For this review, take the finished solid that the model builds, in its own axes (mm). A direction names the side the tool comes from. Give positions to 0.01 mm unless a question says otherwise; leave off trailing zeros. Order: outer loops, then holes, each group sorted by start corner. A loop starts at its lowest first (then second) coordinate and runs counter-clockwise, first axis right, second up. Notation, with made-up numbers: (32, -16.75) - (51, -16.75) arc R8 cw to (51, -10.75) - close; hole circle Ø3 at (60.25, 38). An arc over 180 degrees is marked (long way). One line per item, written item: value.
```python
from build123d import *

# Parameters (mm, degrees)
F2_R     = 0.5
F3_SIZE  = 0.5
F5_DEPTH = 2.38


# Not quite as in the source:
# - a fillet or chamfer that OpenCascade refuses, or shapes differently, is made with other operations: its cross-section is extruded or revolved along the edge and cut away or added


with BuildPart() as f1:
    # F0 (on Front) → F1 (revolve)
    with BuildSketch(Plane.XZ):
        Polygon((-3, 0), (0, 0), (0, 18), (-1.5, 18.8660254038), (-1.5, 24), (-5, 24), (-5, 20), (-3, 20), (-3, 14.25), (-2.5, 14), (-3, 13.75), align=None)
    revolve(axis=Axis((0, 0, 18.332445994), (0, 0, 1)))

    # F2
    f2_edges = [f1.edges().sort_by_distance(p)[0] for p in [
        (5, 0, 24),
    ]]
    fillet(f2_edges, radius=F2_R)

    # F3
    f3_edges = [f1.edges().sort_by_distance(p)[0] for p in [
        (3, 0, 0),
    ]]
    chamfer(f3_edges, length=F3_SIZE)

    # F4 (on face) → F5 (cut)
    with BuildSketch(Plane.XY.offset(24)):
        Polygon((-1.443375673, -2.5), (1.443375673, -2.5), (2.8867513459, 0), (1.443375673, 2.5), (-1.443375673, 2.5), (-2.8867513459, 0), align=None)
    extrude(amount=-F5_DEPTH, mode=Mode.SUBTRACT)

    # F6: chamfer of 1 x 1.7320508076 on 1 edges, made by hand


with BuildPart() as f6_tool2:
    # F6_s3 → F6_t4 (revolve)
    with BuildSketch(Plane.XZ):
        Polygon((-3.2320508076, 21.62), (-1.5, 20.62), (-1.5, 21.62), align=None)
    revolve(axis=Axis((0, 0, 21.62), (0, 0, 1)))

    split(bisect_by=Plane(origin=(-2.1650635095, 1.25, 0), x_dir=(0, 0, 1), z_dir=(0.8660254038, -0.5, 0)), keep=Keep.TOP)

    split(bisect_by=Plane.XZ.offset(-2.5), keep=Keep.TOP)

    split(bisect_by=Plane(origin=(2.1650635095, 1.25, 0), x_dir=(0, 0, 1), z_dir=(-0.8660254038, -0.5, 0)), keep=Keep.TOP)

    split(bisect_by=Plane(origin=(2.1650635095, -1.25, 0), x_dir=(0, 0, 1), z_dir=(-0.8660254038, 0.5, 0)), keep=Keep.TOP)

    split(bisect_by=Plane.XZ.offset(2.5), keep=Keep.BOTTOM)

    split(bisect_by=Plane(origin=(-2.1650635095, -1.25, 0), x_dir=(0, 0, 1), z_dir=(0.8660254038, 0.5, 0)), keep=Keep.TOP)


with BuildPart() as f1_1:
    add(f1.part)

    # F6_t1: cut F6_tool2
    add(f6_tool2.part, mode=Mode.SUBTRACT)


solid = f1_1.part
```
(1) Draft analysis for pull direction Y (two halves, no side actions). For faces 4 (the face through (3, 0, 17)), 5 (the face through (-3.3, -0.1, 20)), 6 (the face through (1.5, -0.07, 19.76)), state which applies: pulls with the +Y half, pulls with the -Y half, needs draft (parallel to the pull), parting line crosses it, or undercut.
Answers below:
face 4: parting line crosses it
face 5: needs draft
face 6: undercut
(2) Machinability: for faces 1 (the face through (0, 2.5, 23)), 2 (the face through (3, 0, 7)), 3 (the face through (2, 2, 24)), which of the approach directions +Z, -Z, +X, -X, +Y, -Y give a long, thin tool a straight path to every point of the face, cutting with its end or side? Answer none if there is none.
Answers below:
face 1: +Z
face 2: -Z
face 3: +Z, +X, -X, +Y, -Y
(3) Wall thickness on line 1 (X direction, y = 0, z = 19.65); line 2 (Y direction, x = 0, z = 20.25): over which ranges is each line inside the solid? List them lowest first. Write a range as from..to.
Answers below:
line 1: x = -3..-1.5, 1.5..3
line 2: y = -5..-1.5, 1.5..5
(4) Take a section at A-A (z = 11.5). Write out the cut boundary in (x, y), then the cut area to 3 significant figures.
Answers below:
outline: circle Ø6 at (0, 0)
area: 28.3 mm^2
(5) For P1, Ø0.8, axis at x = 0.5, z = 23, coming from the -Y side; P2, Ø3, axis at x = 3.5, z = 15.5, coming from the -Y side; P3, Ø6, axis at x = 3, z = 5, coming from the +Y side; P4, Ø2, axis at y = -3, z = 18, coming from the +X side, all flat-tipped, find the tip position at first contact; note any pin that passes through.
Answers below:
P1: stops at y = -5
P2: stops at y = -2.24
P3: stops at y = 3
P4: stops at x = 2.24
